```python
from build123d import *

# Parameters (mm, degrees)
SKETCH1_R           = 29
BOSS_EXTRUDE1_DEPTH = 22
SKETCH1_5_R         = 1
BOSS_EXTRUDE2_DEPTH = 3
CUT_EXTRUDE1_START  = 22
SKETCH1_6_R         = 1.725
CUT_EXTRUDE1_DEPTH  = 3


with BuildPart() as part:
    # Sketch1 → Boss-Extrude1 (new body)
    with BuildSketch(Plane(origin=(0, 0, 0), x_dir=(1, 0, 0), z_dir=(0, 1, 0))):
        with Locations(Location((0, 0, 0), (0, 0, 270))):
            Circle(SKETCH1_R)
        with BuildLine():
            ThreePointArc((9.414065195, 25.305639223), (-13.5, 23.382685902), (-26.622359024, 4.5))
            ThreePointArc((-26.622359024, 4.5), (-26.120735258, 3.279582529), (-25.143996734, 2.392437072))
            ThreePointArc((-25.143996734, 2.392437072), (-23.75, 0), (-25.143996734, -2.392437072))
            ThreePointArc((-25.143996734, -2.392437072), (-26.120735258, -3.279582529), (-26.622359024, -4.5))
            ThreePointArc((-26.622359024, -4.5), (-13.5, -23.382685902), (9.414065195, -25.305639223))
            ThreePointArc((9.414065195, -25.305639223), (10.220165845, -24.261011563), (10.500087086, -22.971558461))
            ThreePointArc((10.500087086, -22.971558461), (11.875, -20.56810334), (14.643909648, -20.579121389))
            ThreePointArc((14.643909648, -20.579121389), (15.900569413, -20.981429034), (17.208293829, -20.805639223))
            ThreePointArc((17.208293829, -20.805639223), (27, 0), (17.208293829, 20.805639223))
            ThreePointArc((17.208293829, 20.805639223), (15.900569413, 20.981429034), (14.643909648, 20.579121389))
            ThreePointArc((14.643909648, 20.579121389), (11.875, 20.56810334), (10.500087086, 22.971558461))
            ThreePointArc((10.500087086, 22.971558461), (10.220165845, 24.261011563), (9.414065195, 25.305639223))
        make_face(mode=Mode.SUBTRACT)
    extrude(amount=BOSS_EXTRUDE1_DEPTH)

    # Sketch1<5> → Boss-Extrude2 (add)
    with BuildSketch(Plane(origin=(0, 0, 0), x_dir=(1, 0, 0), z_dir=(0, 1, 0))):
        with BuildLine():
            ThreePointArc((-26.622359024, -4.5), (-26.120735258, -3.279582529), (-25.143996734, -2.392437072))
            ThreePointArc((-25.143996734, -2.392437072), (-23.75, 0), (-25.143996734, 2.392437072))
            ThreePointArc((-25.143996734, 2.392437072), (-26.120735258, 3.279582529), (-26.622359024, 4.5))
            ThreePointArc((-26.622359024, 4.5), (-13.5, 23.382685902), (9.414065195, 25.305639223))
            ThreePointArc((9.414065195, 25.305639223), (10.220165845, 24.261011563), (10.500087086, 22.971558461))
            ThreePointArc((10.500087086, 22.971558461), (11.875, 20.56810334), (14.643909648, 20.579121389))
            ThreePointArc((14.643909648, 20.579121389), (15.900569413, 20.981429034), (17.208293829, 20.805639223))
            ThreePointArc((17.208293829, 20.805639223), (27, 0), (17.208293829, -20.805639223))
            ThreePointArc((17.208293829, -20.805639223), (15.900569413, -20.981429034), (14.643909648, -20.579121389))
            ThreePointArc((14.643909648, -20.579121389), (11.875, -20.56810334), (10.500087086, -22.971558461))
            ThreePointArc((10.500087086, -22.971558461), (10.220165845, -24.261011563), (9.414065195, -25.305639223))
            ThreePointArc((9.414065195, -25.305639223), (-13.5, -23.382685902), (-26.622359024, -4.5))
        make_face()
        with Locations(Location((0, 15, 0), (0, 0, 270))):
            Circle(SKETCH1_5_R, mode=Mode.SUBTRACT)
        with Locations(Location((15, 0, 0), (0, 0, 270))):
            Circle(SKETCH1_5_R, mode=Mode.SUBTRACT)
        with Locations(Location((0, -15, 0), (0, 0, 270))):
            Circle(SKETCH1_5_R, mode=Mode.SUBTRACT)
        with Locations(Location((-15, 0, 0), (0, 0, 270))):
            Circle(SKETCH1_5_R, mode=Mode.SUBTRACT)
    extrude(amount=BOSS_EXTRUDE2_DEPTH)

    # Sketch1<6> → Cut-Extrude1 (cut)
    with BuildSketch(Plane(origin=(0, 0, 0), x_dir=(1, 0, 0), z_dir=(0, 1, 0)).offset(CUT_EXTRUDE1_START)):
        with Locations(Location((13.25, 22.9496732, 0), (0, 0, 270))):
            Circle(SKETCH1_6_R)
        with Locations(Location((13.25, -22.9496732, 0), (0, 0, 270))):
            Circle(SKETCH1_6_R)
        with Locations(Location((-26.5, 0, 0), (0, 0, 270))):
            Circle(SKETCH1_6_R)
    extrude(amount=-CUT_EXTRUDE1_DEPTH, mode=Mode.SUBTRACT)


solid = part.part
```
Could you check a few things on this model? Use its own coordinates, in mm. A direction names the side the tool comes from. Round coordinates to 2 decimals unless told otherwise and drop trailing zeros. Loops run counter-clockwise (first coordinate to the right, second up) from the corner with the lowest first, then second, coordinate; pieces in that order, holes last. Notation, with made-up numbers: M -32,6 L 15,6 A35 ccw 15,38 Z; hole C 28.25,32.25 d6. An arc over 180 degrees is marked long. Write item = value, one per line.
1. I need wall thicknesses on probe 1 along X at (y, z) = (0.7, 0); probe 2 along Y at (x, z) = (-6, 23); probe 3 along Z at (x, y) = (-18, 16.75). Which ranges of each line are inside material? Lowest first, please.
Results below:
probe_1 = -29 to -16, -14 to 14, 16 to 29
probe_2 = 0 to 3
probe_3 = -22.74 to -20.12, 20.12 to 22.74
2. Which directions (+Z, -Z, +X, -X, +Y, -Y) give clear straight access to the entire face, cutting with the end or side of a thin tool? Please do faces 4 (the face through (-16, 1, 0)), 5 (the face through (-13.787, 12.367, 23.215)).
Results below:
face_4 = +Y, -Y
face_5 = +Y
3. Thinking about a two-plate mould opening in Z: for faces 1 (the face through (11, 22, -22)), 2 (the face through (10.2, 12.4, 24.3)), 3 (the face through (-11.107, 10.846, 26.789)), which applies, +Z half, -Z half, draft (parallel to the pull), parting line (faces both ways), or undercut?
Results below:
face_1 = draft
face_2 = undercut
face_3 = parting line
4. Will these pins go through, and if not, where does the flat tip stop? P1, Ø10, axis at y = 7, z = 18.5, coming from the +X side; P2, Ø2.5, axis at x = -15, z = 0, coming from the +Y side; P3, Ø1.2, axis at x = 0, z = -15, coming from the -Y side; P4, Ø3, axis at x = -26.5, z = 0, coming from the +Y side.
Results below:
P1 = 25.67
P2 = 3
P3 = through
P4 = 19
5. I want a section at D-D, the plane y = 11.25. Write out the boundary of the cut face in (x, z).
Results below:
outline = C 0,0 d58; hole M -26.62,-4.5 A27 ccw 9.41,-25.31 A3 ccw 10.5,-22.97 A2.75 cw 14.64,-20.58 A3 ccw 17.21,-20.81 A27 ccw 17.21,20.81 A3 ccw 14.64,20.58 A2.75 cw 10.5,22.97 A3 ccw 9.41,25.31 A27 ccw -26.62,4.5 A3 ccw -25.14,2.39 A2.75 cw -25.14,-2.39 A3 ccw Z
6. I want a section at C-C, the plane x = 0. Write out the boundary of the cut face in (y, z).
Results below:
outline = M 0,-29 L 22,-29 L 22,-27 L 3,-27 L 3,-16 L 0,-16 Z; M 0,-14 L 3,-14 L 3,14 L 0,14 Z; M 0,16 L 3,16 L 3,27 L 22,27 L 22,29 L 0,29 Z
7. I want a section at A-A, the plane z = 0. Write out the boundary of the cut face in (x, y) (3 decimals), and give its area (3 significant figures).
Results below:
outline = M -29,0 L -16,0 L -16,3 L -23.75,3 L -23.75,22 L -24.775,22 L -24.775,19 L -28.225,19 L -28.225,22 L -29,22 Z; M -14,0 L 14,0 L 14,3 L -14,3 Z; M 16,0 L 29,0 L 29,22 L 27,22 L 27,3 L 16,3 Z
area = 289 mm²
8. I want a section at B-B, the plane x = -15. Write out the boundary of the cut face in (y, z), and give its area (3 significant figures).
Results below:
outline = M 0,-24.82 L 22,-24.82 L 22,-22.45 L 3,-22.45 L 3,-1 L 0,-1 Z; M 0,1 L 3,1 L 3,22.45 L 22,22.45 L 22,24.82 L 0,24.82 Z
area = 233 mm²
